Print and shaded views of the part. All mm, measured from the part's lowest x, y and z. A direction names the side the tool comes from. Round coordinates to 2 decimals unless told otherwise and drop trailing zeros. Loops run counter-clockwise (first coordinate to the right, second up) from the corner with the lowest first, then second, coordinate; pieces in that order, holes last. Notation, with made-up numbers: (-8.5, 27.25) -> (34.5, 27.25) arc R12 cw to (34.5, 50.25) -> close; hole circle Ø3 at (-15.5, 22). An arc over 180 degrees is marked (long way). Use a Markdown table: item, result.
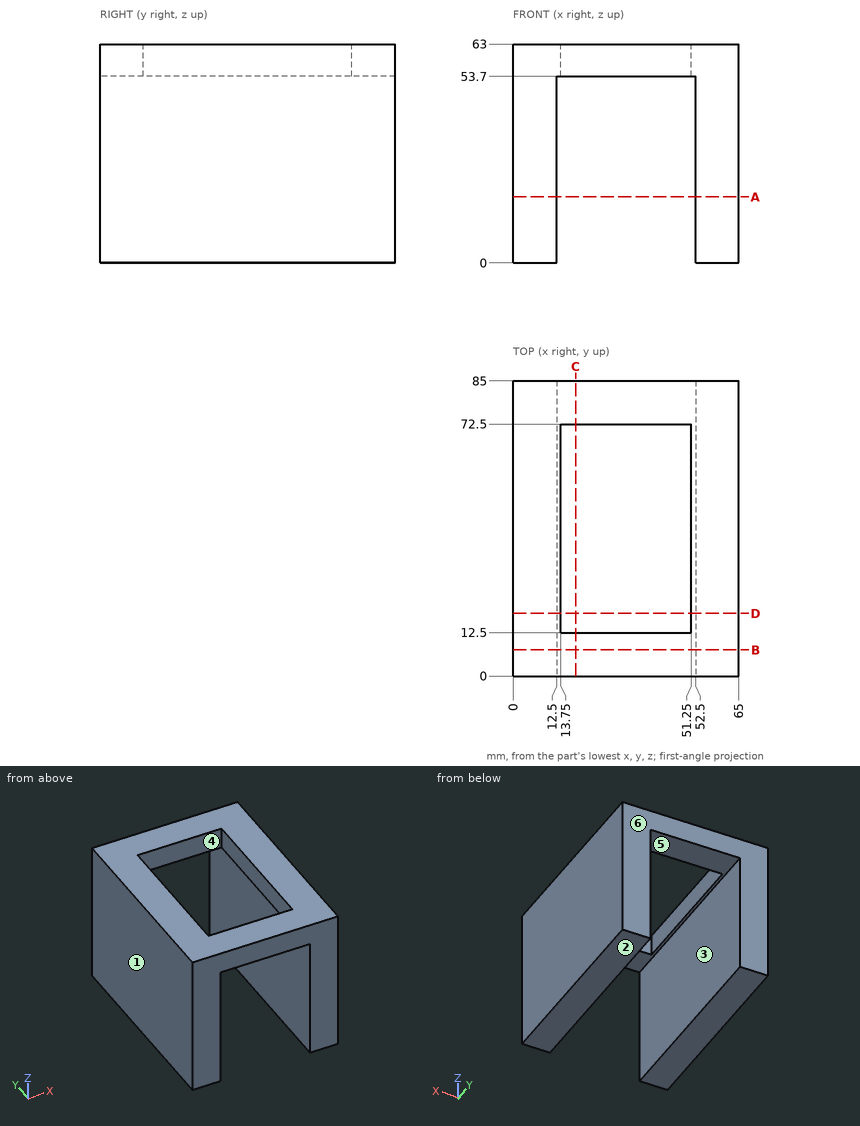
Q1. Tool access for the marked faces 4, 5 and 6: list every direction of +Z, -Z, +X, -X, +Y, -Y with a clear straight run to the whole face (end or side of a thin tool).
Results list:
| item | result |
|---|---|
| face 4 | +Z, -Z |
| face 5 | -Z, +Y, -Y |
| face 6 | +Z, -Z, +X, -X, +Y |
Q2. Band-saw the part on A-A, the plane z = 19. Give the cut face in (x, y).
Results list:
| item | result |
|---|---|
| outline | (0, 0) -> (12.5, 0) -> (12.5, 85) -> (0, 85) -> close; (52.5, 0) -> (65, 0) -> (65, 85) -> (52.5, 85) -> close |
Q3. Band-saw the part on C-C, the plane x = 18. Give the cut face in (y, z).
Results list:
| item | result |
|---|---|
| outline | (0, 53.7) -> (12.5, 53.7) -> (12.5, 63) -> (0, 63) -> close; (72.5, 53.7) -> (85, 53.7) -> (85, 63) -> (72.5, 63) -> close |
Q4. Drill centre lines: L1, parallel to X at y = 67.5, z = 24.5; L2, parallel to X at y = 18, z = 56; L3, parallel to Y at x = 32, z = 57. Where is each one in solid material? Low to high. Write a range as from..to.
Results list:
| item | result |
|---|---|
| L1 | x = 0..12.5, 52.5..65 |
| L2 | x = 0..13.75, 51.25..65 |
| L3 | y = 0..12.5, 72.5..85 |
Q5. Band-saw the part on D-D, the plane y = 18. Give the cut face in (x, z), plus the area to 3 significant figures.
Results list:
| item | result |
|---|---|
| outline | (0, 0) -> (12.5, 0) -> (12.5, 53.7) -> (13.75, 53.7) -> (13.75, 63) -> (0, 63) -> close; (51.25, 53.7) -> (52.5, 53.7) -> (52.5, 0) -> (65, 0) -> (65, 63) -> (51.25, 63) -> close |
| area | 1,600 mm² |
Q6. Band-saw the part on B-B, the plane y = 7.5. Give the cut face in (x, z).
Results list:
| item | result |
|---|---|
| outline | (0, 0) -> (12.5, 0) -> (12.5, 53.7) -> (52.5, 53.7) -> (52.5, 0) -> (65, 0) -> (65, 63) -> (0, 63) -> close |
Q7. Flat gauge pin, fed straight in: pin 1 (20 mm diameter, centred on x = 30.5, y = 55, fed in from -Z) (3 decimals). Where does the tip first touch, or does it go through?
Results list:
| item | result |
|---|---|
| pin 1 | passes through |
Q8. Pull direction X, two halves, no side cores. Call the marked faces 1, 2 and 3: released by +X, released by -X, zero draft, split by the parting line, or undercut.
Results list:
| item | result |
|---|---|
| face 1 | released by -X |
| face 2 | zero draft |
| face 3 | undercut |
